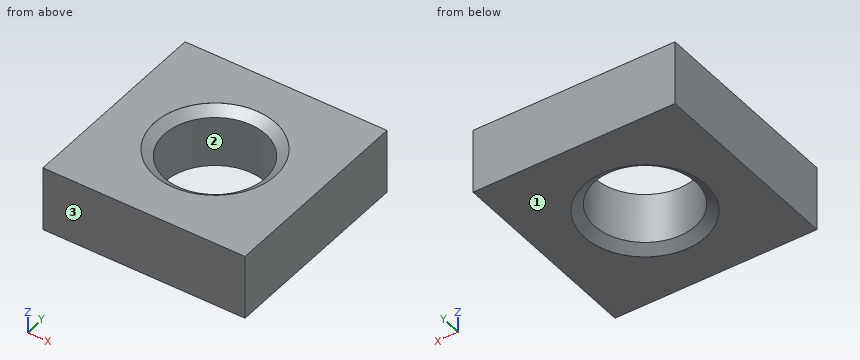
```python
from build123d import *

# Parameters (mm, degrees)
BASENUT_START = -3.2
BASENUTSKE_W  = 10
BASENUTSKE_H  = 10
BASENUTSKE_R  = 2.5
BASENUT_DEPTH = 3.2


with BuildPart() as part:
    # BaseNutSke → BaseNut (new body)
    with BuildSketch(Plane.XY.offset(BASENUT_START)):
        Rectangle(BASENUTSKE_W, BASENUTSKE_H)
        Circle(BASENUTSKE_R, mode=Mode.SUBTRACT)
    extrude(amount=BASENUT_DEPTH)

    # EndChamferSketch → EndChamfer (revolve, cut)
    with BuildSketch(Plane(origin=(0, 0, 0), x_dir=(0, 0, -1), z_dir=(1, 0, 0))):
        Polygon((3.191, 3), (2.805885854, 2.45), (3.201, 2.45), (3.201, 3), align=None)
        Polygon((-0.002, 3), (0.008, 3), (0.393114146, 2.45), (-0.002, 2.45), align=None)
    revolve(axis=Axis((0, 0, -25.037505729), (0, 0, -1)), mode=Mode.SUBTRACT)


solid = part.part
```
Geometry: final body of the model. Coordinates: model frame, mm. Face numbers are marked on the shaded views. Coordinates: 2 decimals unless noted, no trailing zeros. Order: outer loops, then holes, each group sorted by start corner. A loop starts at its lowest first (then second) coordinate and runs counter-clockwise, first axis right, second up. Notation, with made-up numbers: (-12.5, 6) - (-7.5, 6) arc R31 ccw to (-7.5, 41) - close; hole circle Ø11 at (35, 75). An arc over 180 degrees is marked (long way). Return JSON: item names as keys, results as strings. Group by question number.
1. Cut plane C-C (z = -0.7). Output: boundary loops of the cut face in (x, y), plus the area to 3 significant figures.
2. Pull-direction query (Y, two-part tool) for the marked faces 1, 2 and 3; classes: pulls with the +Y half, pulls with the -Y half, needs draft (parallel to the pull), parting line crosses it, or undercut.
3. Material intervals for line 1 along X through (y, z) = (0, -1); line 2 along X through (y, z) = (2, -2.2), sorted ascending. Write a range as [from, to].
Resolved:
{
 "1": {"outline": "(-5, -5) - (5, -5) - (5, 5) - (-5, 5) - close; hole circle Ø5 at (0, 0)", "area": "80.4 mm²"},
 "2": {"face 1": "needs draft", "face 2": "undercut", "face 3": "pulls with the -Y half"},
 "3": {"line 1": "x = [-5, -2.5], [2.5, 5]", "line 2": "x = [-5, -1.5], [1.5, 5]"}
}
